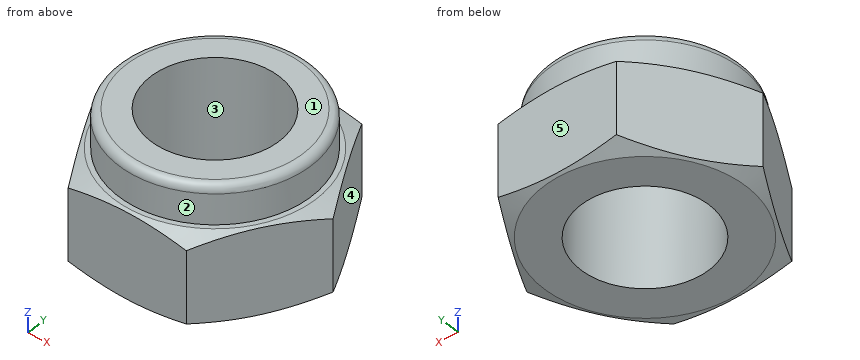
from build123d import *

# Parameters (mm, degrees)
SKETCH007_R  = 4
PAD004_DEPTH = 5.5


with BuildPart() as part:
    # Sketch007 → Pad004 (new body)
    with BuildSketch(Plane.XY):
        Polygon((7.5055534995, 0), (3.7527767497, 6.5), (-3.7527767497, 6.5), (-7.5055534995, 0), (-3.7527767497, -6.5), (3.7527767497, -6.5), align=None)
        Circle(SKETCH007_R, mode=Mode.SUBTRACT)
    extrude(amount=PAD004_DEPTH)

    # Sketch008 → Revolution (revolve)
    with BuildSketch(Plane.XZ):
        with BuildLine():
            Line((4, 5.5), (6, 5.5))
            Line((6, 5.5), (6, 7.4))
            ThreePointArc((6, 7.4), (5.8535533906, 7.7535533906), (5.5, 7.9))
            Line((5.5, 7.9), (4, 7.9))
            Line((4, 7.9), (4, 5.5))
        make_face()
    revolve(axis=Axis((0, 0, 0), (0, 0, 1)))

    # Sketch009 → Groove001 (revolve, cut)
    with BuildSketch(Plane.XZ):
        Polygon((7.5055534995, 5.5), (6.3055534995, 5.5), (7.5055534995, 5), align=None)
        Polygon((7.5055534995, 0), (6.3055534995, 0), (7.5055534995, 0.5), align=None)
    revolve(axis=Axis((0, 0, 0), (0, 0, 1)), mode=Mode.SUBTRACT)


solid = part.part
Read the model definition and answer for the solid it produces. Units are mm, in the model's axes. Face numbers are marked on the shaded views. A direction names the side the tool comes from. Give positions to 0.01 mm unless a question says otherwise; leave off trailing zeros. Loops run counter-clockwise (first coordinate to the right, second up) from the corner with the lowest first, then second, coordinate; pieces in that order, holes last. Notation, with made-up numbers: (41, 68.25) - (76, 68.25) arc R24 cw to (76, 92.25) - close; hole circle Ø9 at (68.25, -13.75). An arc over 180 degrees is marked (long way). Answer as CSV lines item,"result". Start each with the question number.
1) Straight lines are drawn through the part: L1, parallel to Y at x = 0, z = 4.5; L2, parallel to Y at x = 0, z = 6; L3, parallel to X at y = 3, z = 1.5. For each, find the intervals that lie inside material, in ascending order. Write a range as from..to.
2) Determine the mould class of the marked faces 3, 4 and 5 for opening direction X: released by +X, released by -X, zero draft, split by the parting line, or undercut.
3) Which of the six approach directions +Z, -Z, +X, -X, +Y, -Y give full straight-line access (tool end or side, diameter ignored) to the marked faces 1 and 2?
4) Find section A-A (x = 0). Write down the section's boundary in (y, z), then the cut area to 3 significant figures.
5) Find section B-B (z = 1.25). Write down the section's boundary in (x, y).
6) Each of these flat-tipped pins is pushed along its axis until it touches: pin 1 Ø1.5 at (y, z) = (4.5, 6) entering from -X; pin 2 Ø1 at (x, z) = (3.5, 7) entering from +Y; pin 3 Ø6.5 at (x, y) = (0, 0) entering from -Z. Where does it stop, or does it pass through?
Findings below:
1,L1,"-6.5..-4, 4..6.5"
1,L2,"-6..-4, 4..6"
1,L3,"-5.77..-2.65, 2.65..5.77"
2,face 3,"undercut"
2,face 4,"released by +X"
2,face 5,"zero draft"
3,face 1,"+Z, +X, -X, +Y, -Y"
3,face 2,"+Z"
4,outline,"(-6.5, 0.08) - (-6.31, 0) - (-4, 0) - (-4, 7.9) - (-5.5, 7.9) arc R0.5 ccw to (-6, 7.4) - (-6, 5.5) - (-6.31, 5.5) - (-6.5, 5.42) - close; (4, 0) - (6.31, 0) - (6.5, 0.08) - (6.5, 5.42) - (6.31, 5.5) - (6, 5.5) - (6, 7.4) arc R0.5 ccw to (5.5, 7.9) - (4, 7.9) - close"
4,area,"37.0 mm^2"
5,outline,"(-7.51, 0) - (-3.75, -6.5) - (3.75, -6.5) - (7.51, 0) - (3.75, 6.5) - (-3.75, 6.5) - close; hole circle Ø8 at (0, 0)"
6,pin 1,"x = -5.16"
6,pin 2,"y = 5.2"
6,pin 3,"through"
